from build123d import *

# Parameters (mm, degrees)
SKETCH2_W                      = 140
SKETCH2_H                      = 38.89
BOSS_EXTRUDE1_DEPTH            = 4
M2X0_4_TAPPED_HOLE1_AT_2_COUNT = 2
M2X0_4_TAPPED_HOLE1_AT_2_PITCH = 10
SKETCH6_W                      = 120
SKETCH6_H                      = 20
CUT_EXTRUDE1_DEPTH             = 5
SKETCH8_W                      = 35
SKETCH8_H                      = 2.29
SKETCH8_W_2                    = 10
BOSS_EXTRUDE2_DEPTH            = 4
SKETCH9_W                      = 25
SKETCH9_H                      = 2.29
CUT_EXTRUDE3_DEPTH             = 5
SKETCH10_W                     = 140
SKETCH10_H                     = 4
BOSS_EXTRUDE3_DEPTH            = 4
SKETCH11_W                     = 140
SKETCH11_H                     = 3.97
CUT_EXTRUDE4_DEPTH             = 10
CUT_EXTRUDE5_DEPTH             = 5
CUT_EXTRUDE6_DEPTH             = 10


with BuildPart() as part:
    # Sketch2 → Boss-Extrude1 (new body)
    with BuildSketch(Plane(origin=(0, 0, 0), x_dir=(1, 0, 0), z_dir=(0, 1, 0))):
        Rectangle(SKETCH2_W, SKETCH2_H)
    extrude(amount=BOSS_EXTRUDE1_DEPTH)

    # Sketch4 → M2x0.4 Tapped Hole1 (revolve, cut)
    with BuildSketch(Plane(origin=(-70, 2, 4.445), x_dir=(0, 0, 1), z_dir=(0, 1, 0))):
        Polygon((0, 0), (0, 18.480688495), (0.8, 18), (0.8, 0), align=None)
    m2x0_4_tapped_hole1 = revolve(axis=Axis((-76.35, 2, 4.445), (1, 0, 0)), mode=Mode.SUBTRACT)

    # M2x0.4 Tapped Hole1 at 2: M2x0.4 Tapped Hole1 ×2
    with Locations(*[(0, 0, i * M2X0_4_TAPPED_HOLE1_AT_2_PITCH) for i in range(1, M2X0_4_TAPPED_HOLE1_AT_2_COUNT)]):
        add(m2x0_4_tapped_hole1, mode=Mode.SUBTRACT)

    # Mirror1: M2x0.4 Tapped Hole1 across plane
    add(m2x0_4_tapped_hole1.mirror(Plane(origin=(0, 0, 0), x_dir=(0, 0, 1), z_dir=(1, 0, 0))), mode=Mode.SUBTRACT)

    # Mirror1 copy 1 sketch → Mirror1 copy 1 (revolve, cut)
    with BuildSketch(Plane(origin=(70, 2, 14.445), x_dir=(0, 0, 1), z_dir=(0, 1, 0))):
        Polygon((0, 0), (0, -18.480688495), (0.8, -18), (0.8, 0), align=None)
    revolve(axis=Axis((76.35, 2, 14.445), (1, 0, 0)), mode=Mode.SUBTRACT)

    # Sketch6 → Cut-Extrude1 (cut, through all)
    with BuildSketch(Plane(origin=(0, 4, 0), x_dir=(1, 0, 0), z_dir=(0, 1, 0))):
        with Locations((0, -9.445)):
            Rectangle(SKETCH6_W, SKETCH6_H)
    extrude(amount=-CUT_EXTRUDE1_DEPTH, mode=Mode.SUBTRACT)

    # Sketch8 → Boss-Extrude2 (add, through all)
    with BuildSketch(Plane(origin=(0, 4, 0), x_dir=(1, 0, 0), z_dir=(0, 1, 0))):
        with Locations((-52.5, -20.59)):
            Rectangle(SKETCH8_W, SKETCH8_H)
        with Locations((65, -20.59)):
            Rectangle(SKETCH8_W_2, SKETCH8_H)
    extrude(amount=-BOSS_EXTRUDE2_DEPTH)

    # Sketch9 → Cut-Extrude3 (cut, through all)
    with BuildSketch(Plane(origin=(0, 4, 0), x_dir=(1, 0, 0), z_dir=(0, 1, 0))):
        with Locations((-47.5, -20.59)):
            Rectangle(SKETCH9_W, SKETCH9_H)
    extrude(amount=-CUT_EXTRUDE3_DEPTH, mode=Mode.SUBTRACT)

    # Sketch10 → Boss-Extrude3 (add, through all)
    with BuildSketch(Plane(origin=(0, 4, 0), x_dir=(1, 0, 0), z_dir=(0, 1, 0))):
        with Locations((0, 21.445)):
            Rectangle(SKETCH10_W, SKETCH10_H)
    extrude(amount=-BOSS_EXTRUDE3_DEPTH)

    # Sketch11 → Cut-Extrude4 (cut)
    with BuildSketch(Plane(origin=(0, 4, 0), x_dir=(1, 0, 0), z_dir=(0, 1, 0))):
        with Locations((0, -19.75)):
            Rectangle(SKETCH11_W, SKETCH11_H)
    extrude(amount=-CUT_EXTRUDE4_DEPTH, mode=Mode.SUBTRACT)

    # Sketch7 → Cut-Extrude5 (cut, through all)
    with BuildSketch(Plane(origin=(0, 4, 0), x_dir=(1, 0, 0), z_dir=(0, 1, 0))):
        with BuildLine():
            Line((-42, 18.055), (-42, 5.055))
            ThreePointArc((-42, 5.055), (-45, 2.055), (-48, 5.055))
            Line((-48, 5.055), (-48, 18.055))
            ThreePointArc((-48, 18.055), (-45, 21.055), (-42, 18.055))
        make_face()
        with BuildLine():
            Line((48, 18.055), (48, 5.055))
            ThreePointArc((48, 5.055), (45, 2.055), (42, 5.055))
            Line((42, 5.055), (42, 18.055))
            ThreePointArc((42, 18.055), (45, 21.055), (48, 18.055))
        make_face()
    extrude(amount=-CUT_EXTRUDE5_DEPTH, mode=Mode.SUBTRACT)

    # Sketch13 → Cut-Extrude6 (cut)
    with BuildSketch(Plane(origin=(0, 4, 0), x_dir=(1, 0, 0), z_dir=(0, 1, 0))):
        with BuildLine():
            Line((-15, 0.555), (15, 0.555))
            ThreePointArc((15, 0.555), (0, 15.555), (-15, 0.555))
        make_face()
    extrude(amount=-CUT_EXTRUDE6_DEPTH, mode=Mode.SUBTRACT)


solid = part.part
CAD build for the part. Positions are in the model's coordinates, mm. A direction names the side the tool comes from. Round coordinates to 2 decimals unless told otherwise and drop trailing zeros. Loops run counter-clockwise (first coordinate to the right, second up) from the corner with the lowest first, then second, coordinate; pieces in that order, holes last.
(1) Two-plate mould, pull along Z, no slides. Class faces 4 (the flat face through (-42, 2, -12)), 5 (the cylindrical face through (-44.934, 2.028, -2.056)), 6 (the flat face through (-1, 0, -17)), 7 (the flat face through (65, 2, 17.765)): +Z half, -Z half, draft (parallel to the pull), parting line (faces both ways), or undercut.
(2) Wall check: line 1 along Z through (x, y) = (-64, 2) (3 decimals); line 2 along X through (y, z) = (2.05, -18); line 3 along X through (y, z) = (3.6, 11). Give the ranges that are in metal, low to high.
(3) Cut at A-A (y = 2). State how many separate pieces and enclosed holes the cut face has, plus the area to 3 significant figures.
(4) Cut at B-B (z = 6.5). Give the cut face in (x, y), plus the area to 3 significant figures.
(5) Drop flat-ended pins along their axis: pin 1 (1.2 mm diameter, centred on x = 42.5, y = 2.5, fed in from +Z) (3 decimals); pin 2 (2 mm diameter, centred on y = 2, z = 4.445, fed in from +X). Give the stop position or say it passes through.
(6) Which spindle directions (+Z, -Z, +X, -X, +Y, -Y) get a long thin tool onto all of the face, cutting with end or side? Do faces 1 (the flat face through (37, 2, -0.555)), 2 (the flat face through (48, 2, -12)), 3 (the flat face through (-70, 2, -3)). Say none if no direction does.
(7) Cut at C-C (x = 45). Give the cut face in (y, z) (3 decimals), plus the area to 3 significant figures.
(8) Cut at D-D (z = -11). Give the cut face in (x, y), plus the area to 3 significant figures.
Findings below:
1. face 4: undercut
1. face 5: undercut
1. face 6: draft
1. face 7: +Z half
2. line 1: z = -23.445 to 3.645, 5.245 to 13.645, 15.245 to 17.765
2. line 2: x = -70 to -48, -42 to 42, 48 to 70
2. line 3: x = -70 to -60, 60 to 70
3. separate pieces: 5
3. enclosed holes: 2
3. area: 2,940 mm2
4. outline: (-70, 0) - (-60, 0) - (-60, 4) - (-70, 4) - close; (60, 0) - (70, 0) - (70, 4) - (60, 4) - close
4. area: 80.0 mm2
5. pin 1: stops at z = -0.555
5. pin 2: stops at x = 70
6. face 1: +Z, +Y, -Y
6. face 2: +Y, -Y
6. face 3: +Z, -Z, -X, +Y, -Y
7. outline: (0, -23.445) - (4, -23.445) - (4, -21.055) - (0, -21.055) - close; (0, -2.055) - (4, -2.055) - (4, -0.555) - (0, -0.555) - close
7. area: 15.6 mm2
8. outline: (-70, 0) - (-48, 0) - (-48, 4) - (-70, 4) - close; (-42, 0) - (-10.77, 0) - (-10.77, 4) - (-42, 4) - close; (10.77, 0) - (42, 0) - (42, 4) - (10.77, 4) - close; (48, 0) - (70, 0) - (70, 4) - (48, 4) - close
8. area: 426 mm2
